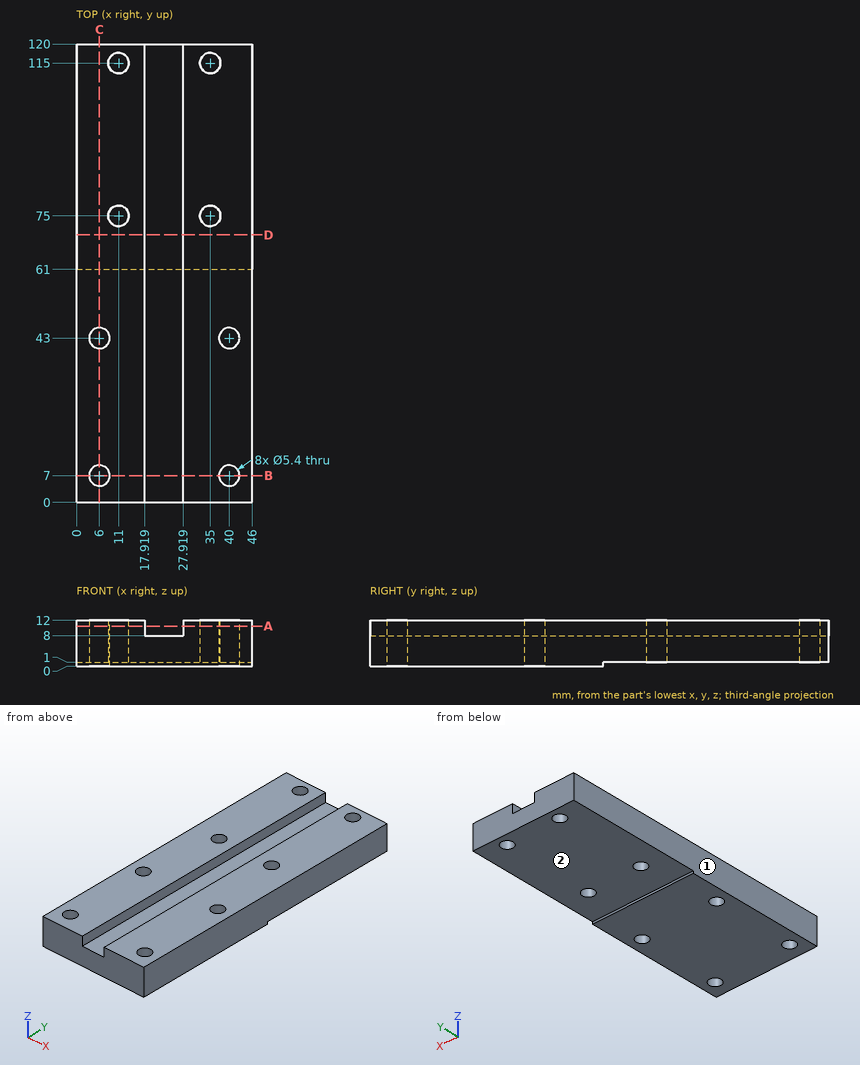
Check sheet for the drawn part. Datum: minimum x, y, z corner. Units: mm. A direction names the side the tool comes from. Round coordinates to 2 decimals unless told otherwise and drop trailing zeros. Order: outer loops, then holes, each group sorted by start corner. A loop starts at its lowest first (then second) coordinate and runs counter-clockwise, first axis right, second up. Notation, with made-up numbers: (-15, 66.5) -> (2, 66.5) arc R33 ccw to (2, 99.5) -> close; hole circle Ø11 at (-18.5, -33). An arc over 180 degrees is marked (long way). Return JSON: item names as keys, results as strings. Group by question number.
Q1. Section check D-D, the plane y = 70. Record the boundary of the cut face in (x, z).
Q2. Material ranges on probe 1 along Y at (x, z) = (11, 6.75); probe 2 along X at (y, z) = (115, 9); probe 3 along Y at (x, z) = (6, 4), recorded low to high. Write a range as from..to.
Q3. Section check B-B, the plane y = 7. Record the boundary of the cut face in (x, z).
Q4. Section check A-A, the plane z = 10.5. Count the separate pieces of the cut face and the enclosed holes in it, plus the area to 3 significant figures.
Q5. Gauge pin test, flat ends, axial feed: pin 1 (3 mm diameter, centred on x = 40, y = 43, fed in from -Z); pin 2 (23 mm diameter, centred on x = 28.5, y = 82, fed in from -Z); pin 3 (8 mm diameter, centred on x = 22.5, y = 64, fed in from +Z). Record the tip position at first contact, or that the pin passes through.
Q6. Tool access check on the marked faces 1 and 2. Record the directions out of +Z, -Z, +X, -X, +Y, -Y that give a thin tool (end or side, any length) a straight path to the whole face; none if there is none.
Q7. Section check C-C, the plane x = 6. Record the boundary of the cut face in (y, z), plus the area to 3 significant figures.
Numbers:
{
 "1": {"outline": "(0, 1) -> (46, 1) -> (46, 12) -> (27.92, 12) -> (27.92, 8) -> (17.92, 8) -> (17.92, 12) -> (0, 12) -> close"},
 "2": {"probe 1": "0..72.3, 77.7..112.3, 117.7..120", "probe 2": "0..8.3, 13.7..17.92, 27.92..32.3, 37.7..46", "probe 3": "0..4.3, 9.7..40.3, 45.7..120"},
 "3": {"outline": "(0, 0) -> (3.3, 0) -> (3.3, 12) -> (0, 12) -> close; (8.7, 0) -> (37.3, 0) -> (37.3, 12) -> (27.92, 12) -> (27.92, 8) -> (17.92, 8) -> (17.92, 12) -> (8.7, 12) -> close; (42.7, 0) -> (46, 0) -> (46, 12) -> (42.7, 12) -> close"},
 "4": {"separate pieces": "2", "enclosed holes": "8", "area": "4,140 mm^2"},
 "5": {"pin 1": "through", "pin 2": "z = 1", "pin 3": "z = 8"},
 "6": {"face 1": "+Z, -Z, -X, +Y, -Y", "face 2": "-Z, +X, -X, +Y"},
 "7": {"outline": "(0, 0) -> (4.3, 0) -> (4.3, 12) -> (0, 12) -> close; (9.7, 0) -> (40.3, 0) -> (40.3, 12) -> (9.7, 12) -> close; (45.7, 0) -> (61, 0) -> (61, 1) -> (120, 1) -> (120, 12) -> (45.7, 12) -> close", "area": "1,250 mm^2"}
}
